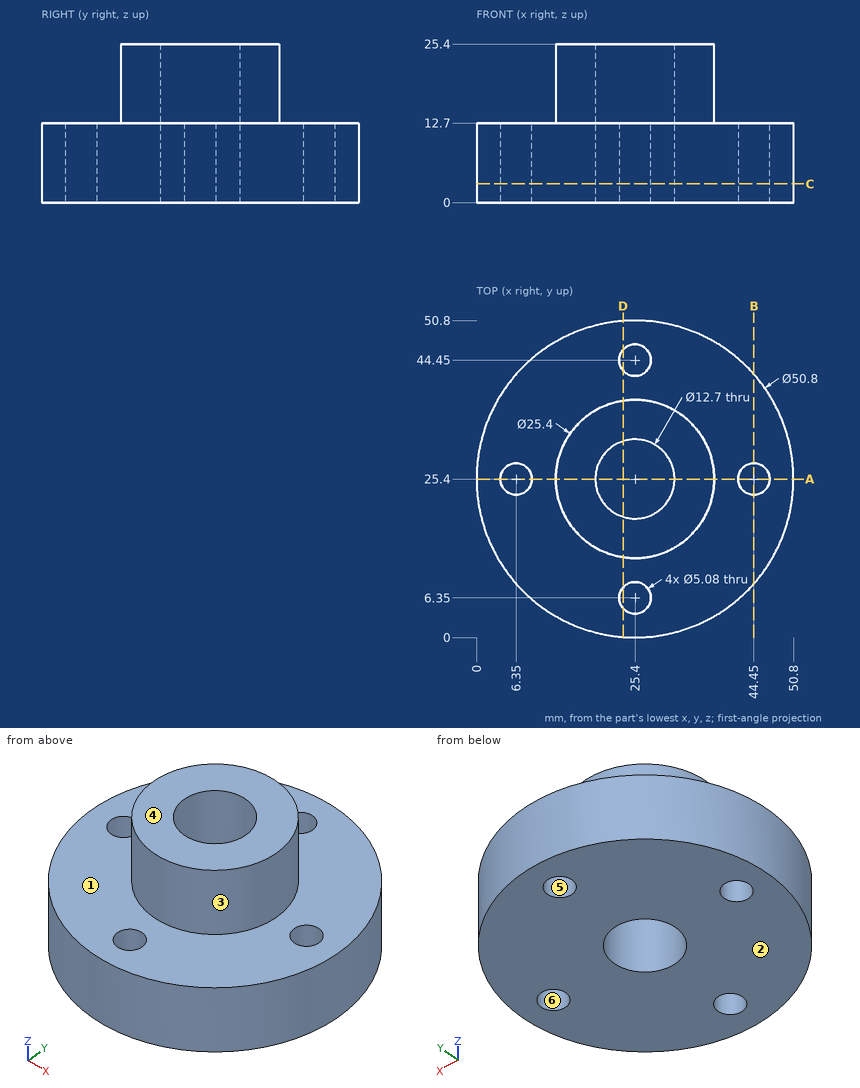
Geometry: see drawing. Coordinates: mm, zero at the bounding-box minimum. A direction names the side the tool comes from. Coordinates: 2 decimals unless noted, no trailing zeros. Order: outer loops, then holes, each group sorted by start corner. A loop starts at its lowest first (then second) coordinate and runs counter-clockwise, first axis right, second up. Notation, with made-up numbers: M -32,70 L -14,70 A20 cw -14,103 Z; hole C 37,27 d6. An arc over 180 degrees is marked long. Answer as CSV lines item,"result".
1. Pull-direction query (X, two-part tool) for the marked faces 3, 4, 5 and 6; classes: released by +X, released by -X, zero draft, split by the parting line, or undercut.
Reported:
face 3,"split by the parting line"
face 4,"zero draft"
face 5,"undercut"
face 6,"undercut"
2. Section D-D (x = 23.5). Return the cut outline in (y, z), then the cut area to 3 significant figures.
Reported:
outline,"M 0.07,0 L 4.66,0 L 4.66,12.7 L 0.07,12.7 Z; M 8.04,0 L 19.34,0 L 19.34,25.4 L 12.84,25.4 L 12.84,12.7 L 8.04,12.7 Z; M 31.46,0 L 42.76,0 L 42.76,12.7 L 37.96,12.7 L 37.96,25.4 L 31.46,25.4 Z; M 46.14,0 L 50.73,0 L 50.73,12.7 L 46.14,12.7 Z"
area,"569 mm2"
3. First-contact query: P1, Ø10, axis at x = 12, z = 12.5, coming from the +Y side; P2, Ø4.5, axis at x = 25.4, y = 6.35, coming from the -Z side; P3, Ø16.5, axis at x = 25.4, y = 25.4, coming from the -Z side; P4, Ø8, axis at y = 38.5, z = 10.5, coming from the +X side. Flat tips, straight axial feed; report the tip coordinate or a pass-through.
Reported:
P1,"y = 49.37"
P2,"through"
P3,"z = 0"
P4,"x = 49.11"
4. Section B-B (x = 44.45). Return the cut outline in (y, z).
Reported:
outline,"M 8.6,0 L 22.86,0 L 22.86,12.7 L 8.6,12.7 Z; M 27.94,0 L 42.2,0 L 42.2,12.7 L 27.94,12.7 Z"
5. Material intervals for line 1 (Y direction, x = 25.4, z = 3.5); line 2 (Y direction, x = 25.4, z = 16.25); line 3 (Z direction, x = 44, y = 30), sorted ascending. Write a range as from..to.
Reported:
line 1,"0..3.81, 8.89..19.05, 31.75..41.91, 46.99..50.8"
line 2,"12.7..19.05, 31.75..38.1"
line 3,"0..12.7"
6. Section A-A (y = 25.4). Return the cut outline in (x, z).
Reported:
outline,"M 0,0 L 3.81,0 L 3.81,12.7 L 0,12.7 Z; M 8.89,0 L 19.05,0 L 19.05,25.4 L 12.7,25.4 L 12.7,12.7 L 8.89,12.7 Z; M 31.75,0 L 41.91,0 L 41.91,12.7 L 38.1,12.7 L 38.1,25.4 L 31.75,25.4 Z; M 46.99,0 L 50.8,0 L 50.8,12.7 L 46.99,12.7 Z"
7. Access query for the marked faces 1 and 2. Directions: +Z, -Z, +X, -X, +Y, -Y. A direction counts if a zero-diameter tool reaches every point of the face in a straight line with its end or side. Return the directions, or none.
Reported:
face 1,"+Z"
face 2,"-Z, +X, -X, +Y, -Y"
8. Section C-C (z = 3). Return the cut outline in (x, y).
Reported:
outline,"C 25.4,25.4 d50.8; hole C 6.35,25.4 d5.08; hole C 25.4,25.4 d12.7; hole C 25.4,6.35 d5.08; hole C 25.4,44.45 d5.08; hole C 44.45,25.4 d5.08"
